Design review of the part built by this model. Coordinates are the model's own, in mm. Face numbers are marked on the shaded views. A direction names the side the tool comes from. Give positions to 0.01 mm unless a question says otherwise; leave off trailing zeros. Loops run counter-clockwise (first coordinate to the right, second up) from the corner with the lowest first, then second, coordinate; pieces in that order, holes last. Notation, with made-up numbers: M 3,-14.75 L 51,-14.75 A32 cw 51,13.25 Z; hole C 53,40 d3. An arc over 180 degrees is marked long. Use CSV: the item, a comma, the result in double quotes.
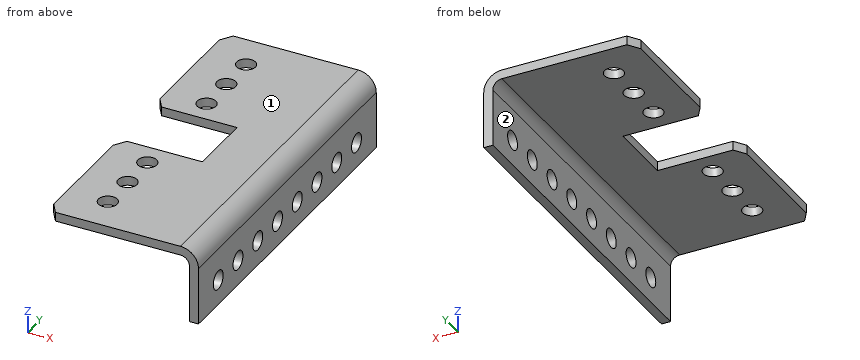
Autodesk Inventor part; units mm, degrees
ref_plane "YZ Plane" through (0, 0, 0) normal (1, 0, 0) x (0, 1, 0)
ref_plane "XZ Plane" through (0, 0, 0) normal (0, 1, 0) x (-1, 0, 0)
ref_plane "XY Plane" through (0, 0, 0) normal (0, 0, 1) x (1, 0, 0)
sketch "Sketch1" plane through (0, 0, 0) normal (0, 0, 1) x (1, 0, 0)
  line L0 (0, 46.0375) -> (-2.644, 42.0764)
  line L1 (-2.644, 42.0764) -> (-2.644, 3.9764)
  line L2 (-2.644, 3.9764) -> (0, 0)
  line L3 (0, 46.0375) -> (25.4, 46.0375)
  line L4 (25.4, 46.0375) -> (25.4, 68.2625)
  line L5 (25.4, 57.15) -> (26.8908, 57.15)
  line L6 (0, 68.2625) -> (-2.644, 72.2236)
  line L7 (-2.644, 72.2236) -> (-2.644, 110.3236)
  line L8 (-2.644, 110.3236) -> (0, 114.3)
  line L9 (0, 68.2625) -> (25.4, 68.2625)
  line L10 (25.4, 68.2625) -> (25.4, 46.0375)
  line L11 (48.156, 114.3) -> (0, 114.3)
  line L12 (48.156, 114.3) -> (48.156, 0)
  line L13 (0, 0) -> (48.156, 0)
  line L14 (218.3648, 132.2525) -> (215.7208, 128.2914)
  line L15 (215.7208, 128.2914) -> (215.7208, 90.1914)
  line L16 (215.7208, 90.1914) -> (218.3648, 86.215)
  line L17 (218.3648, 132.2525) -> (234.2398, 132.2525)
  line L18 (218.3648, 154.4775) -> (215.7208, 158.4387)
  line L19 (215.7208, 158.4387) -> (215.7208, 196.5387)
  line L20 (215.7208, 196.5387) -> (218.3648, 200.515)
  line L21 (218.3648, 154.4775) -> (234.2398, 154.4775)
  line L22 (253.8208, 200.515) -> (218.3648, 200.515)
  line L23 (253.8208, 200.515) -> (253.8208, 86.215)
  line L24 (218.3648, 86.215) -> (253.8208, 86.215)
  line L25 (379.0105, 160.3375) -> (376.3665, 156.3764)
  line L26 (376.3665, 156.3764) -> (376.3665, 118.2764)
  line L27 (376.3665, 118.2764) -> (379.0105, 114.3)
  line L28 (379.0105, 160.3375) -> (398.0605, 160.3375)
  line L29 (398.0605, 160.3375) -> (398.0605, 182.5625)
  line L30 (398.0605, 171.45) -> (393.2013, 171.45)
  line L31 (379.0105, 182.5625) -> (376.3665, 186.5236)
  line L32 (376.3665, 186.5236) -> (376.3665, 224.6236)
  line L33 (376.3665, 224.6236) -> (379.0105, 228.6)
  line L34 (379.0105, 182.5625) -> (398.0605, 182.5625)
  line L35 (398.0605, 182.5625) -> (398.0605, 160.3375)
  line L36 (414.4665, 228.6) -> (379.0105, 228.6)
  line L37 (414.4665, 228.6) -> (414.4665, 114.3)
  line L38 (379.0105, 114.3) -> (414.4665, 114.3)
  line L39 (237.4148, 151.3025) -> (237.4148, 135.4275)
  arc A0 (237.4148, 151.3025) -> (234.2398, 154.4775) centre (234.2398, 151.3025) ccw
  arc A1 (234.2398, 132.2525) -> (237.4148, 135.4275) centre (234.2398, 135.4275) ccw
  line L40 (0, 114.3) -> (48.156, 114.3)
  line L41 (48.156, 114.3) -> (48.156, 0)
  line L42 (48.156, 0) -> (0, 0)
  line L43 (0, 0) -> (-2.644, 3.9764)
  line L44 (-2.644, 3.9764) -> (-2.644, 42.0764)
  line L45 (-2.644, 42.0764) -> (0, 46.0375)
  line L46 (0, 46.0375) -> (25.4, 46.0375)
  line L47 (25.4, 46.0375) -> (25.4, 68.2625)
  line L48 (25.4, 68.2625) -> (0, 68.2625)
  line L49 (0, 68.2625) -> (-2.644, 72.2236)
  line L50 (-2.644, 72.2236) -> (-2.644, 110.3236)
  line L51 (-2.644, 110.3236) -> (0, 114.3)
  dimension "d1" = 46.0375
  dimension "d5" = 38.1
  dimension "d6" = 4.7625
  dimension "d8" = 4.7752
  dimension "d9" = 25.4
  dimension "d12" = 22.225
  dimension "d14" = 114.3
  dimension "d15" = 22.756
  dimension "d16" = 21.2652
  dimension "d26" = 46.0375
  dimension "d27" = 38.1
  dimension "d28" = 4.7625
  dimension "d29" = 4.7752
  dimension "d30" = 19.05
  dimension "d31" = 22.225
  dimension "d32" = 114.3
  dimension "d33" = 16.406
  dimension "d34" = 21.2652
  dimension "d35" = 3.175
extrude "Plate1" add sketch "Sketch1" along normal blind 3.048 contours L3 L4 L9 L6 L7 L8 L11 L12 L13 L2 L1 L0
sketch "Sketch5" plane through (45.108, 0, 3.048) normal (1, 0, 0) x (0, 1, 0)
  line L0 (114.3, 0) -> (0, 0)
  line L1 (0, 0) -> (0, -25.4)
  line L2 (0, -25.4) -> (114.3, -25.4)
  line L3 (114.3, -25.4) -> (114.3, 0)
edge flange "Flange1" height 25.4 angle 90 thickness 3.048 bend radius 3.048 thickness toward (1, 0, 0) relief tear relief width 3.048 relief depth 1.524 edges at (48.156, 57.15, 0) wall of the first edge with corners at (45.108, 114.3, 3.048) (45.108, 0, 3.048) (45.108, 0, -22.352) (45.108, 114.3, -22.352)
bend "Bend2"
corner "Corner1"
sketch "Sketch6" plane through (0, 0, 0) normal (0, 0, -1) x (-1, 0, 0)
  line L0 (0, 114.3) -> (-42.06, 114.3)
  line L1 (0, 0) -> (-42.06, 0)
  point P0 (-10.9909, 101.6)
  point P1 (-10.9909, 88.9)
  point P2 (-10.9909, 76.2)
  point P3 (-10.9909, 38.1)
  point P4 (-10.9909, 25.4)
  point P5 (-10.9909, 12.7)
  dimension "d91" = 12.7
  dimension "d92" = 12.7
  dimension "d93" = 12.7
  dimension "d94" = 12.7
  dimension "d95" = 12.7
  dimension "d96" = 12.7
hole "Hole3" at (10.9909, 101.6, 0) at (10.9909, 88.9, 0) at (10.9909, 76.2, 0) at (10.9909, 38.1, 0) at (10.9909, 25.4, 0) at (10.9909, 12.7, 0) direction (0, 0, 1) diameter 6.35 depth 3.048 tip angle 118
sketch "Sketch7" plane through (48.156, 0, -22.352) normal (1, 0, 0) x (0, 0, -1)
  line L0 (0, 0) -> (-19.304, 0)
  point P0 (-22.352, 0)
  point P1 (-8.5162, 101.6)
  point P2 (-8.5162, 88.9)
  point P3 (-8.5162, 76.2)
  point P4 (-8.5162, 63.5)
  point P5 (-8.5162, 50.8)
  point P6 (-8.5162, 38.1)
  point P7 (-8.5162, 25.4)
  point P8 (-8.5162, 12.7)
  dimension "d104" = 12.7
  dimension "d105" = 12.7
  dimension "d106" = 12.7
  dimension "d107" = 12.7
  dimension "d108" = 12.7
  dimension "d109" = 12.7
  dimension "d110" = 12.7
  dimension "d111" = 12.7
hole "Hole4" at (48.156, 88.9, -13.8358) at (48.156, 101.6, -13.8358) at (48.156, 76.2, -13.8358) at (48.156, 63.5, -13.8358) at (48.156, 50.8, -13.8358) at (48.156, 25.4, -13.8358) at (48.156, 38.1, -13.8358) at (48.156, 12.7, -13.8358) direction (-1, 0, 0) diameter 6.35 depth 3.048 tip angle 118
equation "\"d102\" = Thickness"
equation "\"d117\" = Thickness"
equation "\"d81\" = BendReliefWidth"
equation "\"d82\" = BendReliefDepth"
equation "\"d83\" = MinimumRemnant"
equation "\"d84\" = BendRadius"
equation "\"d87\" = BendRadius"
equation "\"d88\" = CornerReliefSize"
equation "\"d89\" = GapSize"
equation "\"d90\" = JacobiRadiusSize"
equation "\"BendRadius\" = Thickness"
equation "\"BendReliefWidth\" = Thickness"
equation "\"BendReliefDepth\" = 0.5 * Thickness"
equation "\"CornerReliefSize\" = 4 * Thickness"
equation "\"MinimumRemnant\" = 2 * Thickness"
equation "\"TransitionRadius\" = BendRadius"
equation "\"JacobiRadiusSize\" = BendRadius"
equation "\"GapSize\" = Thickness"
equation "\"d36\" = BendRadius"
properties part number "Transmission bracket"
(1) We need section D-D on y = 63.5. State the section outline as (x, z) points, then the cut area to 3 significant figures.
A:
outline,"M 25.4,0 L 42.06,0 A3.05 cw 45.11,-3.05 L 45.11,-10.66 L 48.16,-10.66 L 48.16,-3.05 A6.1 ccw 42.06,3.05 L 25.4,3.05 Z; M 45.11,-22.35 L 48.16,-22.35 L 48.16,-17.01 L 45.11,-17.01 Z"
area,"112 mm²"
(2) We need section A-A on x = 18.5. State the section outline as (y, z) points, then the cut area to 3 significant figures.
A:
outline,"M 0,0 L 46.04,0 L 46.04,3.05 L 0,3.05 Z; M 68.26,0 L 114.3,0 L 114.3,3.05 L 68.26,3.05 Z"
area,"281 mm²"
(3) Machinability: for the marked faces 1 and 2, which of the approach directions +Z, -Z, +X, -X, +Y, -Y give a long, thin tool a straight path to every point of the face, cutting with its end or side? Answer none if there is none.
A:
face 1,"+Z, +X, -X, +Y, -Y"
face 2,"-Z, -X, +Y, -Y"
(4) We need section C-C on y = 19.5. State the section outline as (x, z) points.
A:
outline,"M -2.64,0 L 42.06,0 A3.05 cw 45.11,-3.05 L 45.11,-22.35 L 48.16,-22.35 L 48.16,-3.05 A6.1 ccw 42.06,3.05 L -2.64,3.05 Z"
(5) Clearance check with flat-ended pins moving along their axes: P1, Ø10, axis at y = 88.9, z = -13.84, coming from the -X side; P2, Ø13.5, axis at x = 16, y = 34.5, coming from the -Z side; P3, Ø1.5, axis at y = 61.5, z = 1.5, coming from the -X side. State where each tip first meets the part, or that it passes through.
A:
P1,"x = 45.11"
P2,"z = 0"
P3,"x = 25.4"
(6) We need section B-B on y = 88.9. State the section outline as (x, z) points.
A:
outline,"M -2.64,0 L 7.82,0 L 7.82,3.05 L -2.64,3.05 Z; M 14.17,0 L 42.06,0 A3.05 cw 45.11,-3.05 L 45.11,-10.66 L 48.16,-10.66 L 48.16,-3.05 A6.1 ccw 42.06,3.05 L 14.17,3.05 Z; M 45.11,-22.35 L 48.16,-22.35 L 48.16,-17.01 L 45.11,-17.01 Z"
(7) Wall thickness on line 1 along X through (y, z) = (58.5, -5.25); line 2 along Z through (x, y) = (41, 44.5); line 3 along X through (y, z) = (12.7, 2.3): over which ranges is each line inside the solid? List them lowest first. Write a range as [from, to].
A:
line 1,"[45.11, 48.16]"
line 2,"[0, 3.05]"
line 3,"[-2.64, 7.82], [14.17, 44.99]"
